Part model, mm, in its own coordinate system. A direction names the side the tool comes from. Give positions to 0.01 mm unless a question says otherwise; leave off trailing zeros. Write each loop counter-clockwise with the first axis right and the second up, starting at its lowest first coordinate (ties: lowest second). Pieces come first, ordered by that corner, then holes. Notation, with made-up numbers: M -17,-31 L 1,-31 A3 ccw 1,-27 Z; hole C 21,47 d4. An arc over 180 degrees is marked long. Answer as CSV lines item,"result". Start each with the question number.
Item 1: 3-axis set-ups, long thin cutter, end or side, ignore diameter. For faces 1 (the flat face through (-78.35, 4, 3)), 2 (the flat face through (22, 37.194, -5)): which of +Z, -Z, +X, -X, +Y, -Y reach the whole face in a straight line?
Item 2: Band-saw the part on C-C, the plane y = 0.5. List the corners of the cut face in (x, z), then the cut area to 3 significant figures.
Item 3: Wall check: L1, parallel to Y at x = -43.5, z = -0.25; L2, parallel to Z at x = 11, y = -19. Give the ranges that are in metal, low to high. Write a range as from..to.
Item 4: Band-saw the part on B-B, the plane z = -2. List the corners of the cut face in (x, y).
Item 5: Band-saw the part on A-A, the plane x = 25.5. List the corners of the cut face in (y, z), then the cut area to 3 significant figures.
Item 6: Pin check, flat tip, straight feed: pin 1 (8 mm diameter, centred on x = 28, y = 22, fed in from -Z). Stop position of the tip, or through.
from build123d import *

# Parameters (mm, degrees)
SKETCH1_W           = 197.4
SKETCH1_H           = 85.209366976
BOSS_EXTRUDE1_DEPTH = 6
BOSS_EXTRUDE2_DEPTH = 10


with BuildPart() as part:
    # Sketch1 → Boss-Extrude1 (new body)
    with BuildSketch(Plane.XY):
        with Locations((20.35, 4.589716511)):
            Rectangle(SKETCH1_W, SKETCH1_H)
    extrude(amount=BOSS_EXTRUDE1_DEPTH)

    # Sketch2 → Boss-Extrude2 (add)
    with BuildSketch(Plane(origin=(0, 47.194399999, 0), x_dir=(1, 0, 0), z_dir=(0, 1, 0))):
        Polygon((-78.35, 0), (-68.35, 10), (109.05, 10), (119.05, 0), (119.05, -6), (-78.35, -6), align=None)
    extrude(amount=-BOSS_EXTRUDE2_DEPTH)


solid = part.part
Output:
1,face 1,"+Z, -Z, -X, +Y, -Y"
1,face 2,"-Z, +X, -X, -Y"
2,outline,"M -78.35,0 L 119.05,0 L 119.05,6 L -78.35,6 Z"
2,area,"1,180 mm²"
3,L1,"37.19..47.19"
3,L2,"0..6"
4,outline,"M -76.35,37.19 L 117.05,37.19 L 117.05,47.19 L -76.35,47.19 Z"
5,outline,"M -38.01,0 L 37.19,0 L 37.19,-10 L 47.19,-10 L 47.19,6 L -38.01,6 Z"
5,area,"611 mm²"
6,pin 1,"z = 0"
